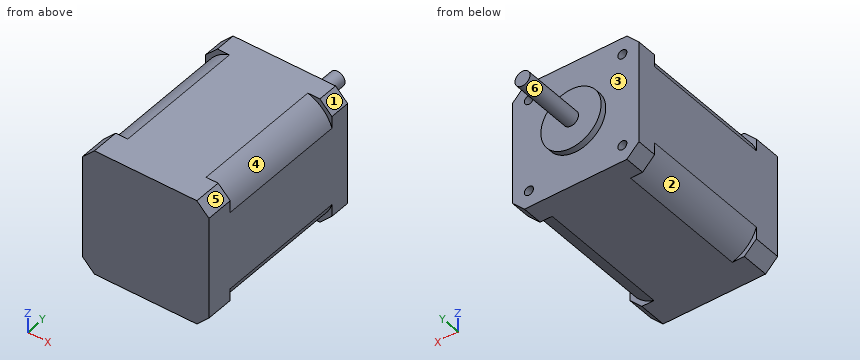
Autodesk Inventor part; units mm, degrees
ref_plane "YZ Plane" through (0, 0, 0) normal (1, 0, 0) x (0, 1, 0)
ref_plane "XZ Plane" through (0, 0, 0) normal (0, 1, 0) x (-1, 0, 0)
ref_plane "XY Plane" through (0, 0, 0) normal (0, 0, 1) x (1, 0, 0)
sketch "Sketch1" plane through (0, 0, 0) normal (0, 1, 0) x (-1, 0, 0)
  line L0 (-21, 21) -> (21, 21)
  line L1 (21, 21) -> (21, -21)
  line L2 (21, -21) -> (-21, -21)
  line L3 (-21, -21) -> (-21, 21)
  line L4 (-21, 21) -> (21, -21) construction
  line L5 (21, 21) -> (-21, -21) construction
  point P0 (0, 0)
  dimension "d0" = 42
  dimension "d1" = 42
extrude "Extrusion1" add sketch "Sketch1" along normal blind 60
sketch "Sketch3" plane through (0, 60, 0) normal (0, 1, 0) x (1, 0, 0)
  circle A0 centre (0, 0) radius 10
  dimension "d4" = 20
extrude "Extrusion2" add sketch "Sketch3" along normal blind 2
sketch "Sketch4" plane through (0, 60, 0) normal (0, 1, 0) x (1, 0, 0)
  circle A0 centre (0, 0) radius 10
  line L0 (-15.5, 15.5) -> (15.5, 15.5)
  line L1 (15.5, 15.5) -> (15.5, -15.5)
  line L2 (15.5, -15.5) -> (-15.5, -15.5)
  line L3 (-15.5, -15.5) -> (-15.5, 15.5)
  line L4 (-15.5, 15.5) -> (15.5, -15.5) construction
  line L5 (15.5, 15.5) -> (-15.5, -15.5) construction
  circle A1 centre (15.5, 15.5) radius 1.5
  circle A2 centre (-15.5, 15.5) radius 1.5
  circle A3 centre (-15.5, -15.5) radius 1.5
  circle A4 centre (15.5, -15.5) radius 1.5
  dimension "d7" = 31
  dimension "d8" = 31
  dimension "d9" = 3
  dimension "d10" = 3
  dimension "d11" = 3
  dimension "d12" = 3
extrude "Extrusion3" cut sketch "Sketch4" against normal blind 10 contours L3 A2 L0 | L0 A2 L3 | A1 L1 L0 | L0 L1 A1 | A3 L2 L3 | L3 L2 A3 | A4 L2 L1 | L1 L2 A4
chamfer "Chamfer1" distance 4 angle 45 4 edges at (-21, 30, -21) (21, 30, -21) (-21, 30, 21) (21, 30, 21)
sketch "Sketch5" plane through (0, 62, 0) normal (0, 1, 0) x (1, 0, 0)
  circle A0 centre (0, 0) radius 10
  circle A1 centre (0, 0) radius 2.5
  dimension "d18" = 5
extrude "Extrusion4" add sketch "Sketch5" along normal blind 21 contours A1
ref_plane "Work Plane1" through (0, 9.2, 0) normal (0, -1, 0) x (1, 0, 0)
sketch "Sketch6" plane through (0, 9.2, 0) normal (0, -1, 0) x (1, 0, 0)
  line L0 (17, 21) -> (21, 17)
  line L1 (17, 21) -> (-17, 21)
  line L2 (-21, 17) -> (-17, 21)
  line L3 (-21, 17) -> (-21, -17)
  line L4 (-17, -21) -> (-21, -17)
  line L5 (-17, -21) -> (17, -21)
  line L6 (21, -17) -> (17, -21)
  line L7 (21, -17) -> (21, 17)
  arc A0 (21, 13) -> (13, 21) centre (9.5, 9.5) ccw
  point P0 (0, 0)
extrude "Extrusion5" cut sketch "Sketch6" against normal blind 44 contours L0 L7 A0 L1
pattern_circular "Circular Pattern1" count 4 over 360 about axis through (0, 62, 0) along (0, 1, 0) of "Extrusion5"
properties part number "stepmotor" material "Rubber"
Geometry: final body of the model. Coordinates: model frame, mm. Face numbers are marked on the shaded views. A direction names the side the tool comes from. Round coordinates to 2 decimals unless told otherwise and drop trailing zeros. Order: outer loops, then holes, each group sorted by start corner. A loop starts at its lowest first (then second) coordinate and runs counter-clockwise, first axis right, second up. Notation, with made-up numbers: (-9, -25.75) -> (4, -25.75) arc R26 ccw to (4, -4.75) -> close; hole circle Ø3 at (-0.5, -10.75). An arc over 180 degrees is marked (long way). Use CSV: the item, a comma, the result in double quotes. Start each with the question number.
1) Section D-D (x = -15.5). Return the cut outline in (y, z).
2) Draft query along Y for the marked faces 1, 2, 3 and 4. Return one class per face: +Y half, -Y half, draft (parallel to the pull), parting line (faces both ways), or undercut.
3) Section A-A (x = 0). Return the cut outline in (y, z).
4) Material intervals for line 1 along Z through (x, y) = (-15.5, 55.75); line 2 along Y through (x, z) = (9, 1.5), sorted ascending. Write a range as from..to.
5) Set-up query: the marked faces 5 and 6. Return all of +Z, -Z, +X, -X, +Y, -Y with unobstructed straight access to the full face (end or side cutting, diameter ignored); none if empty.
6) Section B-B (y = 36.5). Return the cut outline in (x, z), and give its area (3 significant figures).
7) First-contact query: pin 1 Ø1.5 at (x, z) = (-15.5, -15) entering from +Y; pin 2 Ø5 at (x, y) = (9, 62) entering from -Z; pin 3 Ø1.5 at (x, y) = (-3, 69.5) entering from +Z; pin 4 Ø2.5 at (x, z) = (16, -18.5) entering from +Y. Flat tips, straight axial feed; report the tip coordinate or a pass-through.
8) Section C-C (z = 0). Return the cut outline in (x, y).
Returned:
1,outline,"(0, -21) -> (9.2, -21) -> (9.2, -19.92) -> (53.2, -19.92) -> (53.2, -21) -> (60, -21) -> (60, -17) -> (50, -17) -> (50, -14) -> (60, -14) -> (60, 14) -> (50, 14) -> (50, 17) -> (60, 17) -> (60, 21) -> (53.2, 21) -> (53.2, 19.92) -> (9.2, 19.92) -> (9.2, 21) -> (0, 21) -> close"
2,face 1,"draft"
2,face 2,"undercut"
2,face 3,"+Y half"
2,face 4,"undercut"
3,outline,"(0, -21) -> (60, -21) -> (60, -10) -> (62, -10) -> (62, -2.5) -> (83, -2.5) -> (83, 2.5) -> (62, 2.5) -> (62, 10) -> (60, 10) -> (60, 21) -> (0, 21) -> close"
4,line 1,"z = -21..-17, -14..14, 17..21"
4,line 2,"y = 0..62"
5,face 5,"+Z, +X, +Y, -Y"
5,face 6,"+Y"
6,outline,"(-21, -13) arc R12.02 ccw to (-13, -21) -> (13, -21) arc R12.02 ccw to (21, -13) -> (21, 13) arc R12.02 ccw to (13, 21) -> (-13, 21) arc R12.02 ccw to (-21, 13) -> close"
6,area,"1,680 mm²"
7,pin 1,"stops at y = 50"
7,pin 2,"stops at z = -21"
7,pin 3,"stops at z = 1.09"
7,pin 4,"stops at y = 60"
8,outline,"(-21, 0) -> (21, 0) -> (21, 60) -> (10, 60) -> (10, 62) -> (2.5, 62) -> (2.5, 83) -> (-2.5, 83) -> (-2.5, 62) -> (-10, 62) -> (-10, 60) -> (-21, 60) -> close"
